Part model, mm, in its own coordinate system. Coordinates: 2 decimals unless noted, no trailing zeros. Order: outer loops, then holes, each group sorted by start corner. A loop starts at its lowest first (then second) coordinate and runs counter-clockwise, first axis right, second up.
```python
from build123d import *

# Parameters (mm, degrees)
SKETCH1_W           = 1524
SKETCH1_H           = 609.6
BOSS_EXTRUDE1_DEPTH = 38.1
SKETCH2_R           = 19.05
CUT_EXTRUDE1_DEPTH  = 39.1


with BuildPart() as part:
    # Sketch1 → Boss-Extrude1 (new body)
    with BuildSketch(Plane(origin=(0, 0, 0), x_dir=(1, 0, 0), z_dir=(0, 1, 0))):
        Rectangle(SKETCH1_W, SKETCH1_H)
    extrude(amount=-BOSS_EXTRUDE1_DEPTH)

    # Sketch2 → Cut-Extrude1 (cut, through all)
    with BuildSketch(Plane(origin=(0, 0, 0), x_dir=(1, 0, 0), z_dir=(0, 1, 0))):
        with Locations((-152, 0)):
            Circle(SKETCH2_R)
    extrude(amount=-CUT_EXTRUDE1_DEPTH, mode=Mode.SUBTRACT)


solid = part.part
```
(1) Pull direction X, two halves, no side cores. Call faces 1 (the face through (762, -19, 4)), 2 (the face through (-11, 0, -4)), 3 (the face through (-762, -19, 4)), 4 (the face through (-171.03, -18.78, -0.84)): +X half, -X half, draft (parallel to the pull), parting line (faces both ways), or undercut.
(2) Slice it at A-A, the plane z = 0. Give the cut face in (x, y), then the cut area to 3 significant figures.
(3) Slice it at B-B, the plane x = -152. Give the cut face in (y, z).
(4) Probe line 1 (Z direction, x = -152, y = -29); line 2 (X direction, y = -15.5, z = 0); line 3 (X direction, y = -35.5, z = 4). List the from-to ranges inside material, lowest first.
Here are the results:
1. face 1: +X half
1. face 2: draft
1. face 3: -X half
1. face 4: undercut
2. outline: (-762, -38.1) - (-171.05, -38.1) - (-171.05, 0) - (-762, 0) - close; (-132.95, -38.1) - (762, -38.1) - (762, 0) - (-132.95, 0) - close
2. area: 56,600 mm2
3. outline: (-38.1, -304.8) - (0, -304.8) - (0, -19.05) - (-38.1, -19.05) - close; (-38.1, 19.05) - (0, 19.05) - (0, 304.8) - (-38.1, 304.8) - close
4. line 1: z = -304.8 to -19.05, 19.05 to 304.8
4. line 2: x = -762 to -171.05, -132.95 to 762
4. line 3: x = -762 to -170.63, -133.37 to 762
